Model file for the job. Use its own axes, mm. A direction names the side the tool comes from. Give positions to 0.01 mm unless a question says otherwise; leave off trailing zeros. Order: outer loops, then holes, each group sorted by start corner. A loop starts at its lowest first (then second) coordinate and runs counter-clockwise, first axis right, second up. Notation, with made-up numbers: M 39.25,46 L 59.25,46 A18 cw 59.25,66 Z; hole C 20.5,87 d10. An arc over 180 degrees is marked long. Return JSON: item names as keys, results as strings. Group by question number.
1. Slice it at C-C on y = 35.5. List the corners of the cut face in (x, z).
2. Pin check, flat tips, straight feed: pin 1 (1.5 mm diameter, centred on x = 20, y = 20, fed in from -Z); pin 2 (1.1 mm diameter, centred on y = 23.5, z = 88.5, fed in from +X); pin 3 (3 mm diameter, centred on x = 26.5, y = 22, fed in from +Z); pin 4 (6 mm diameter, centred on y = 35, z = 36.5, fed in from -X). Stop position of each tip, or through.
3. 3-axis set-ups, long thin cutter, end or side, ignore diameter. For faces 1 (the face through (0, 20, 9)), 2 (the face through (35, 36, 18)), 3 (the face through (24, 7, 71.2)): which of +Z, -Z, +X, -X, +Y, -Y reach the whole face in a straight line?
4. Wall check: probe 1 along Y at (x, z) = (20, 90); probe 2 along Z at (x, y) = (18, 6.5); probe 3 along Y at (x, z) = (19.5, 50). Give the ranges that are in metal, low to high. Write a range as [from, to].
5. Slice it at A-A on z = 86. List the corners of the cut face in (x, y).
6. Two-plate mould, pull along Y, no slides. Class faces 4 (the face through (40, 20, 9)), 5 (the face through (25.54, 17.7, 73.69)), 6 (the face through (32.06, 32.3, 63.38)): released by +Y, released by -Y, zero draft, split by the parting line, or undercut.
7. Slice it at B-B on z = 67.5. List the corners of the cut face in (x, y), then the cut area to 3 significant figures.
8. Slice it at D-D on z = 38. List the corners of the cut face in (x, y).
from build123d import *

# Parameters (mm, degrees)
SKETCH_1_W               = 40
SKETCH_1_H               = 40
EXTRUDE_1_DEPTH          = 18
SKETCH_2_R               = 20
EXTRUDE_2_DEPTH          = 53.2
SKETCH_3_R               = 13
EXTRUDE_3_DEPTH          = 2
SKETCH_4_R               = 6
EXTRUDE_4_DEPTH          = 1
SKETCH_5_R               = 5
EXTRUDE_5_DEPTH          = 23
CUT_EXTRUDE_1_DEPTH      = 1.8
HOLE_WIZARD_M31_D        = 2.5
HOLE_WIZARD_M31_DEPTH    = 15
HOLE_WIZARD_M31_TIP      = 0.751075774
PATTERN_CIRCULAR_1_COUNT = 4


with BuildPart() as part:
    # Эскиз1 → Бобышка-Вытянуть1 (new body)
    with BuildSketch(Plane.XY):
        with Locations((20, 20)):
            Rectangle(SKETCH_1_W, SKETCH_1_H)
    extrude(amount=EXTRUDE_1_DEPTH)

    # Эскиз2 → Бобышка-Вытянуть2 (add)
    with BuildSketch(Plane.XY.offset(18)):
        with Locations((20, 20)):
            Circle(SKETCH_2_R)
    extrude(amount=EXTRUDE_2_DEPTH)

    # Эскиз3 → Бобышка-Вытянуть3 (add)
    with BuildSketch(Plane.XY.offset(71.2)):
        with Locations((20, 20)):
            Circle(SKETCH_3_R)
    extrude(amount=EXTRUDE_3_DEPTH)

    # Эскиз4 → Бобышка-Вытянуть4 (add)
    with BuildSketch(Plane.XY.offset(73.2)):
        with Locations((20, 20)):
            Circle(SKETCH_4_R)
    extrude(amount=EXTRUDE_4_DEPTH)

    # Эскиз5 → Бобышка-Вытянуть5 (add)
    with BuildSketch(Plane.XY.offset(74.2)):
        with Locations((20, 20)):
            Circle(SKETCH_5_R)
    extrude(amount=EXTRUDE_5_DEPTH)

    # Эскиз9 → Вырез-Вытянуть1 (cut)
    with BuildSketch(Plane(origin=(0, 25, 0), x_dir=(-1, 0, 0), z_dir=(0, -1, 0))):
        with BuildLine():
            Line((-21.068455004, -93.2), (-21.068455004, -78.2))
            ThreePointArc((-21.068455004, -78.2), (-19.568455004, -76.7), (-18.068455004, -78.2))
            Line((-18.068455004, -78.2), (-18.068455004, -93.2))
            ThreePointArc((-18.068455004, -93.2), (-19.568455004, -94.7), (-21.068455004, -93.2))
        make_face()
    extrude(amount=CUT_EXTRUDE_1_DEPTH, mode=Mode.SUBTRACT)

    # Отверстие обработанное метчиком M31
    with Locations(Plane.XY.offset(97.2)):
        with Locations((20, 20)):
            Hole(HOLE_WIZARD_M31_D / 2, depth=HOLE_WIZARD_M31_DEPTH)
            with Locations((0, 0, -(HOLE_WIZARD_M31_DEPTH + HOLE_WIZARD_M31_TIP / 2))):  # 118° drill point
                Cone(0, HOLE_WIZARD_M31_D / 2, HOLE_WIZARD_M31_TIP, mode=Mode.SUBTRACT)

    # Эскиз14 → Отверстие обработанное метчиком M41 (revolve, cut)
    with BuildSketch(Plane(origin=(7.97918472, 32.02081528, 71.2), x_dir=(0, -1, 0), z_dir=(1, 0, 0))):
        Polygon((0, 0), (0, 7.991420021), (1.65, 7), (1.65, 0), align=None)
    hole_wizard_m41 = revolve(axis=Axis((7.97918472, 32.02081528, 77.55), (0, 0, -1)), mode=Mode.SUBTRACT)

    # Круговой массив1: Отверстие обработанное метчиком M41 ×4 about axis
    pattern_circular_1_axis = Axis((20, 20, 0), (0, 0, 1))
    for i in range(1, PATTERN_CIRCULAR_1_COUNT):
        add(hole_wizard_m41.rotate(pattern_circular_1_axis, i * 360 / PATTERN_CIRCULAR_1_COUNT), mode=Mode.SUBTRACT)


solid = part.part
Result:
{
 "1": {"outline": "M 0,0 L 40,0 L 40,18 L 32.64,18 L 32.64,71.2 L 7.36,71.2 L 7.36,18 L 0,18 Z"},
 "2": {"pin 1": "stops at z = 0", "pin 2": "stops at x = 24.04", "pin 3": "stops at z = 74.2", "pin 4": "stops at x = 4"},
 "3": {"face 1": "+Z, -Z, -X, +Y, -Y", "face 2": "+Z, +X, +Y", "face 3": "+Z"},
 "4": {"probe 1": "y = [15, 18.75], [21.25, 23.2]", "probe 2": "z = [0, 71.2]", "probe 3": "y = [0.01, 39.99]"},
 "5": {"outline": "M 18.07,23.2 L 18.07,24.61 A5 ccw long 21.07,24.88 L 21.07,23.2 Z; hole C 20,20 d2.5"},
 "6": {"face 4": "zero draft", "face 5": "split by the parting line", "face 6": "undercut"},
 "7": {"outline": "C 20,20 d40; hole C 7.98,7.98 d3.3; hole C 7.98,32.02 d3.3; hole C 32.02,7.98 d3.3; hole C 32.02,32.02 d3.3", "area": "1,220 mm2"},
 "8": {"outline": "C 20,20 d40"}
}
